from build123d import *

# Parameters (mm, degrees)
SKETCH2_R           = 3.175
SKETCH4_R           = 3.175
BOSS_EXTRUDE1_DEPTH = 12.7
SKETCH5_R           = 3.175
BOSS_EXTRUDE2_DEPTH = 88.9


with BuildPart() as part:
    # Sweep1: sweep along a path in Sketch1
    with BuildLine(Plane.XY) as sweep1_path:
        ThreePointArc((41.275, 0), (34.739755092, 102.430538934), (15.24, 203.2))
    # Sketch2 → Sweep1 (sweep)
    with BuildSketch(Plane(origin=(0, 0, 0), x_dir=(1, 0, 0), z_dir=(0, 1, 0))):
        with Locations((41.275, 0)):
            Circle(SKETCH2_R)
    sweep(path=sweep1_path.line)

    # Sketch4 → Boss-Extrude1 (add)
    with BuildSketch(Plane(origin=(-48.605579352, 186.566514737, 0), x_dir=(0.9676982350284877, 0.25211133636302385, 0), z_dir=(-0.25211133636302385, 0.9676982350284877, 0))):
        with Locations((65.976744651, 0)):
            Circle(SKETCH4_R)
    extrude(amount=BOSS_EXTRUDE1_DEPTH)

    # Sketch5 → Boss-Extrude2 (add)
    with BuildSketch(Plane.XZ):
        with Locations((41.275, 0)):
            Circle(SKETCH5_R)
    extrude(amount=BOSS_EXTRUDE2_DEPTH)


solid = part.part
Read the model definition and answer for the solid it produces. Units are mm, in the model's axes. A direction names the side the tool comes from. Coordinates: 2 decimals unless noted, no trailing zeros. Order: outer loops, then holes, each group sorted by start corner. A loop starts at its lowest first (then second) coordinate and runs counter-clockwise, first axis right, second up. Notation, with made-up numbers: M 69,37.25 L 79,37.25 A31 ccw 79,62.25 Z; hole C 24.5,-15.75 d6. An arc over 180 degrees is marked long. Put each result on its own line as item: value. Start each with the question number.
Item 1: For faces 1 (the face through (41, -88.9, 0)), 2 (the face through (38.1, -43.8, 0.1)), determine the directions among +Z, -Z, +X, -X, +Y, -Y from which every point of the face is accessible in a straight line to the end or side of a thin tool.
Item 2: Given pin 1 Ø2 at (y, z) = (182.5, -1.5) entering from +X; pin 2 Ø3 at (x, y) = (34.5, 139.5) entering from +Z, each flat-ended and moving along its own axis, determine where each tip first touches the part or whether it passes through.
Item 3: Section B-B, the plane y = -62.5 is taken. Determine the outline of the cut face in (x, z) (3 decimals), plus the area to 3 significant figures.
Item 4: Section A-A, the plane z = 0 is taken. Determine the outline of the cut face in (x, y).
Item 5: Consider probe 1 along Z at (x, y) = (41.5, -38); probe 2 along X at (y, z) = (128.5, 1); probe 3 along X at (y, z) = (55, -0.25). Determine where each line is inside the solid, lowest interval first. Write a range as [from, to].
Computed:
1. face 1: +Z, -Z, +X, -X, -Y
1. face 2: -Y
2. pin 1: stops at x = 23.66
2. pin 2: passes through
3. outline: C 41.275,0 d6.35
3. area: 31.7 mm2
4. outline: M 8.97,214.69 L 12.17,202.4 A802.82 cw 38.1,0 L 38.1,-88.9 L 44.45,-88.9 L 44.45,0 A809.17 ccw 18.31,204 L 15.11,216.29 Z
5. probe 1: z = [-3.17, 3.17]
5. probe 2: x = [27.91, 34.02]
5. probe 3: x = [36.22, 42.57]
